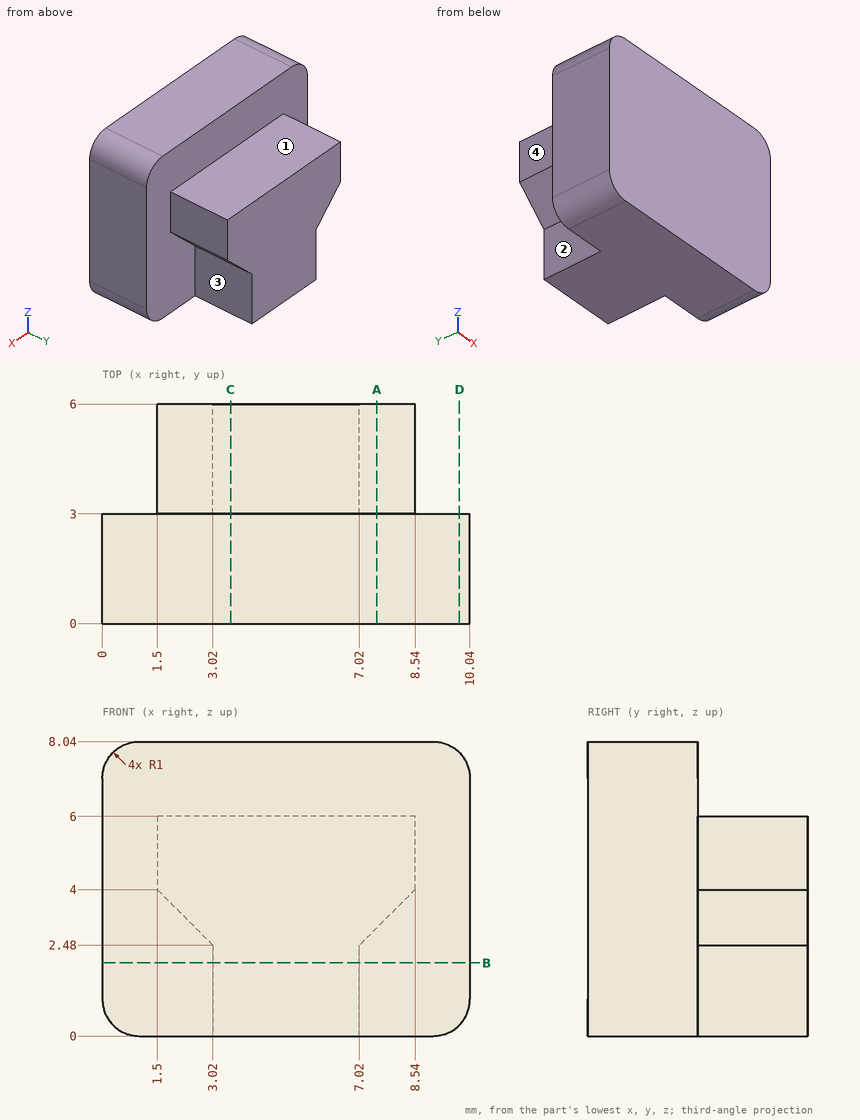
The figure shows three views and two pictorial views of one solid part (mm, origin at its lowest corner). Answer the questions. A direction names the side the tool comes from. Round coordinates to 2 decimals unless told otherwise and drop trailing zeros. Order: outer loops, then holes, each group sorted by start corner. A loop starts at its lowest first (then second) coordinate and runs counter-clockwise, first axis right, second up. Notation, with made-up numbers: M 26,21.5 L 33,21.5 A16 cw 33,34.5 Z; hole C 80,71 d10. An arc over 180 degrees is marked long. Put each result on its own line as item: value. Start each with the question number.
Q1. Section D-D, the plane x = 9.75 is taken. Write down the section's boundary in (y, z), and give its area (3 significant figures).
Q2. Flat-ended cylindrical pins translate along their axes: pin 1 (1 mm diameter, centred on y = 4.5, z = 5.5, fed in from +X); pin 2 (1.5 mm diameter, centred on y = 4.5, z = 2.5, fed in from +X); pin 3 (1.6 mm diameter, centred on y = 4.5, z = 5, fed in from -X). Find the tip coordinate at first contact, or state that the pin passes through.
Q3. Straight lines are drawn through the part: L1, parallel to Y at x = 1.75, z = 1.5; L2, parallel to Z at x = 4.5, y = 4.45; L3, parallel to X at y = 3.95, z = 4.5. For each, find the intervals that lie inside material, in ascending order. Write a range as [from, to].
Q4. Section B-B, the plane z = 2 is taken. Write down the section's boundary in (x, y), and give its area (3 significant figures).
Q5. Section A-A, the plane x = 7.5 is taken. Write down the section's boundary in (y, z).
Q6. Section C-C, the plane x = 3.5 is taken. Write down the section's boundary in (y, z), and give its area (3 significant figures).
Q7. A tool of negligible diameter and unlimited length cuts with its end or side. For the marked faces 1, 2, 3 and 4, from which of +Z, -Z, +X, -X, +Y, -Y can it reach the whole face along a straight path? Write none if from no direction.
Findings below:
1. outline: M 0,0.3 L 3,0.3 L 3,7.74 L 0,7.74 Z
1. area: 22.3 mm^2
2. pin 1: stops at x = 8.54
2. pin 2: stops at x = 7.79
2. pin 3: stops at x = 1.5
3. L1: y = [0, 3]
3. L2: z = [0, 6]
3. L3: x = [1.5, 8.54]
4. outline: M 0,0 L 10.04,0 L 10.04,3 L 7.02,3 L 7.02,6 L 3.02,6 L 3.02,3 L 0,3 Z
4. area: 42.1 mm^2
5. outline: M 0,0 L 3,0 L 3,2.96 L 6,2.96 L 6,6 L 3,6 L 3,8.04 L 0,8.04 Z
6. outline: M 0,0 L 6,0 L 6,6 L 3,6 L 3,8.04 L 0,8.04 Z
6. area: 42.1 mm^2
7. face 1: +Z, +X, -X, +Y
7. face 2: -Z, -X, +Y
7. face 3: -Z, +X, +Y
7. face 4: +Z, -Z, -X, +Y
